from build123d import *

# Parameters (mm, degrees)
F1_DEPTH = 25.4
F4_DEPTH = 15.875


with BuildPart() as f1:
    # F0 (on Front) → F1 (new body)
    with BuildSketch(Plane.XZ):
        with BuildLine():
            Line((862.5024050593, 9.3825748086), (-70.9475949407, 9.3825748086))
            Line((-70.9475949407, 9.3825748086), (-70.9475949407, -66.8174251914))
            ThreePointArc((-70.9475949407, -66.8174251914), (395.7774050593, -16.0174251914), (862.5024050593, -66.8174251914))
            Line((862.5024050593, -66.8174251914), (862.5024050593, 9.3825748086))
        make_face()
    extrude(amount=F1_DEPTH)


with BuildPart() as f4:
    # F3 (on Front) → F4 (new body)
    with BuildSketch(Plane.XZ):
        with BuildLine():
            Line((858.7739929676, 10.8425256968), (-74.6760070324, 10.8425256968))
            Line((-74.6760070324, 10.8425256968), (-74.6760070324, -90.7574743032))
            ThreePointArc((-74.6760070324, -90.7574743032), (392.0489929676, -39.9574743032), (858.7739929676, -90.7574743032))
            Line((858.7739929676, -90.7574743032), (858.7739929676, 10.8425256968))
        make_face()
    extrude(amount=F4_DEPTH)


solid = f4.part
Could you check a few things on this model? Use its own coordinates, in mm. Round coordinates to 2 decimals unless told otherwise and drop trailing zeros. Write each loop counter-clockwise with the first axis right and the second up, starting at its lowest first coordinate (ties: lowest second). Pieces come first, ordered by that corner, then holes. Notation, with made-up numbers: (86, 52.5) - (105, 52.5) arc R18 cw to (105, 64.5) - close; hole circle Ø9 at (-19.75, 10). An arc over 180 degrees is marked (long way). Use a Markdown table: item, result.
Q1. I want a section at C-C (x = 2). List the corners of the cut face in (y, z) for me (3 decimals), plus the area to 3 significant figures.
Output values:
| item | result |
|---|---|
| outline | (-15.875, -75.31) - (0, -75.31) - (0, 10.843) - (-15.875, 10.843) - close |
| area | 1,370 mm2 |
Q2. Thinking about a two-plate mould opening in X: for faces 1 (the flat face through (386, 0, -28)), 2 (the flat face through (-74.676, -8, -39)), 3 (the cylindrical face through (385.463, -7.826, -39.967)), which applies, released by +X, released by -X, zero draft, split by the parting line, or undercut?
Output values:
| item | result |
|---|---|
| face 1 | zero draft |
| face 2 | released by -X |
| face 3 | undercut |
Q3. Please list where these lines run through material, in increasing order: L1, parallel to Z at x = 498.5, y = -9; L2, parallel to Z at x = 800, y = -10.5.
Output values:
| item | result |
|---|---|
| L1 | -42.57 to 10.84 |
| L2 | -78.66 to 10.84 |
Q4. I want a section at B-B (y = -4.5). List the corners of the cut face in (x, z) for me, plus the area to 3 significant figures.
Output values:
| item | result |
|---|---|
| outline | (-74.68, -90.76) arc R2169.42 cw to (858.77, -90.76) - (858.77, 10.84) - (-74.68, 10.84) - close |
| area | 63,200 mm2 |
